Build history of the part. All positions in model axes, mm. A direction names the side the tool comes from. Give positions to 0.01 mm unless a question says otherwise; leave off trailing zeros. Loops run counter-clockwise (first coordinate to the right, second up) from the corner with the lowest first, then second, coordinate; pieces in that order, holes last. Notation, with made-up numbers: (-33, 75) -> (14, 75) arc R22 ccw to (14, 83) -> close; hole circle Ø4 at (44.25, -19.75). An arc over 180 degrees is marked (long way). One line per question, with ' | ' between items. Start each with the question number.
(1) Slice it at C-C, the plane y = 207.5. Write the cut outline in (x, z), then the cut area to 3 significant figures.
(2) Slice it at A-A, the plane x = 58. Write the cut outline in (y, z) (3 decimals), then the cut area to 3 significant figures.
(3) Slice it at B-B, the plane y = 156. Write the cut outline in (x, z) (3 decimals).
(4) Flat gauge pins, fed straight in: pin 1 Ø1.9 at (y, z) = (125, 182) entering from -X; pin 2 Ø10 at (x, y) = (158, 26.5) entering from +Z; pin 3 Ø6 at (x, z) = (95.5, 20) entering from -Y. Where does each tip first touch, or does it go through?
(5) Mould opens along Z. For faces 1 (the face through (90, 223.52, 88)), 2 (the face through (50, 112, 184.15)), 3 (the face through (50, 165.1, 178)) say: pulls with the +Z half, pulls with the -Z half, needs draft (parallel to the pull), parting line crosses it, or undercut.
(6) Drill centre lines: L1, parallel to Y at x = 27, z = 175.5 (3 decimals); L2, parallel to Z at x = 62, y = 190. Where is each one in solid material? Low to high. Write a range as from..to.
(7) 3-axis set-ups, long thin cutter, end or side, ignore diameter. For faces 4 (the face through (172.72, 98, 88)), 5 (the face through (51, 114.3, 178)), 6 (the face through (152.4, 216, 90)): which of +Z, -Z, +X, -X, +Y, -Y reach the whole face in a straight line?
(8) Slice it at D-D, the plane z = 120.5. Write the cut outline in (x, y).
Autodesk Inventor part; units mm, degrees
ref_plane "YZ Plane" through (0, 0, 0) normal (1, 0, 0) x (0, 1, 0)
ref_plane "XZ Plane" through (0, 0, 0) normal (0, 1, 0) x (-1, 0, 0)
ref_plane "XY Plane" through (0, 0, 0) normal (0, 0, 1) x (1, 0, 0)
sketch "Sketch1" plane through (0, 0, 0) normal (0, 0, 1) x (1, 0, 0)
  line L0 (0, 0) -> (177.8, 0)
  line L1 (177.8, 0) -> (177.8, 203.2)
  line L2 (177.8, 203.2) -> (0, 203.2)
  line L3 (0, 203.2) -> (0, 0)
  line L4 (0, 203.2) -> (25.4, 203.2) construction
  line L5 (177.8, 203.2) -> (203.2, 203.2) construction
  line L6 (0, 203.2) -> (177.8, 203.2)
  line L7 (177.8, 203.2) -> (177.8, 228.6)
  line L8 (177.8, 228.6) -> (0, 228.6)
  line L9 (0, 228.6) -> (0, 203.2)
  dimension "d0" = 177.8
  dimension "d1" = 203.2
  dimension "d6" = 177.8
  dimension "d7" = 25.4
extrude "Extrusion1" add sketch "Sketch1" along normal blind 177.8
sketch "Sketch2" plane through (0, 0, 177.8) normal (0, 0, 1) x (1, 0, 0)
  line L0 (177.8, 228.6) -> (0, 228.6)
  line L1 (0, 228.6) -> (177.8, 228.6)
  line L2 (177.8, 228.6) -> (177.8, 203.2)
  line L3 (177.8, 203.2) -> (0, 203.2)
  line L4 (0, 203.2) -> (0, 228.6)
  point P0 (0, 0)
  dimension "d10" = 177.8
  dimension "d11" = 25.4
extrude "Extrusion2" cut sketch "Sketch2" against normal blind 25.4
sketch "Sketch3" plane through (177.8, 0, 0) normal (1, 0, 0) x (0, 0, -1)
  line L0 (0, 0) -> (0, 228.6)
  line L1 (-177.8, 0) -> (-177.8, 203.2)
  line L2 (0, 228.6) -> (-177.8, 228.6)
  line L3 (-177.8, 228.6) -> (-177.8, 203.2)
  line L4 (-177.8, 203.2) -> (0, 203.2)
  line L5 (0, 203.2) -> (0, 228.6)
  dimension "d14" = 177.8
  dimension "d15" = 25.4
extrude "Extrusion3" cut sketch "Sketch3" against normal blind 25.4
sketch "Sketch4" plane through (0, 0, 0) normal (0, 0, -1) x (-1, 0, 0)
  line L0 (0, 228.6) -> (0, 0)
  line L1 (-152.4, 203.2) -> (-177.8, 203.2)
  line L2 (0, 228.6) -> (-177.8, 228.6)
  line L3 (-177.8, 228.6) -> (-177.8, 203.2)
  line L4 (-177.8, 203.2) -> (0, 203.2)
  line L5 (0, 203.2) -> (0, 228.6)
  dimension "d18" = 177.8
  dimension "d19" = 25.4
extrude "Extrusion4" cut sketch "Sketch4" against normal blind 25.4
sketch "Sketch5" plane through (0, 0, 0) normal (-1, 0, 0) x (0, 0, 1)
  line L0 (177.8, 228.6) -> (0, 228.6)
  line L1 (0, 228.6) -> (0, 203.2)
  line L2 (0, 203.2) -> (177.8, 203.2)
  line L3 (177.8, 203.2) -> (177.8, 228.6)
  line L4 (177.8, 203.2) -> (177.8, 0)
  line L5 (25.4, 228.6) -> (152.4, 228.6)
  point P0 (0, 0)
  dimension "d22" = 177.8
  dimension "d23" = 25.4
  dimension "d24" = 0
  dimension "d25" = 0
extrude "Extrusion5" cut sketch "Sketch5" against normal blind 25.4
shell "Shell1" thickness 5.08 removed faces 1 at (59.2667, 0, 59.2667)
sketch "Sketch6" plane through (0, 0, 177.8) normal (0, 0, 1) x (1, 0, 0)
  line L0 (25.4, 165.1) -> (76.2, 165.1)
  line L1 (76.2, 165.1) -> (76.2, 114.3)
  line L2 (76.2, 114.3) -> (25.4, 114.3)
  line L3 (25.4, 114.3) -> (25.4, 165.1)
  line L4 (177.8, 203.2) -> (0, 203.2)
  line L5 (0, 203.2) -> (0, 0)
  line L6 (47.625, 165.1) -> (53.975, 165.1)
  line L7 (53.975, 114.3) -> (47.625, 114.3)
  line L8 (76.2, 142.875) -> (76.2, 136.525)
  line L9 (25.4, 136.525) -> (25.4, 142.875)
  line L10 (47.625, 114.3) -> (47.625, 136.525)
  line L11 (47.625, 142.875) -> (47.625, 165.1)
  line L12 (25.4, 142.875) -> (47.625, 142.875)
  line L13 (53.975, 142.875) -> (76.2, 142.875)
  line L14 (53.975, 165.1) -> (53.975, 142.875)
  line L15 (53.975, 136.525) -> (53.975, 114.3)
  line L16 (76.2, 136.525) -> (53.975, 136.525)
  line L17 (47.625, 136.525) -> (25.4, 136.525)
  line L18 (82.55, 171.45) -> (19.05, 171.45)
  line L19 (19.05, 171.45) -> (19.05, 107.95)
  line L20 (19.05, 107.95) -> (82.55, 107.95)
  line L21 (82.55, 107.95) -> (82.55, 171.45)
  dimension "d29" = 50.8
  dimension "d30" = 50.8
  dimension "d31" = 38.1
  dimension "d32" = 25.4
  dimension "d33" = 6.35
  dimension "d34" = 50.8
  dimension "d36" = 50.8
  dimension "d37" = 6.35
  dimension "d39" = 6.35
extrude "Extrusion6" cut sketch "Sketch6" against normal blind 25.4 contours L0 L11 L12 L3 | L0 L1 L13 L14 | L17 L10 L2 L3 | L1 L2 L15 L16
extrude "Extrusion7" add sketch "Sketch6" along normal blind 6.35
sketch "Sketch7" plane through (0, 0, 177.8) normal (0, 0, 1) x (1, 0, 0)
  line L0 (0, 0) -> (177.8, 0)
  line L1 (76.2, 0) -> (139.7, 0)
  line L2 (139.7, 0) -> (139.7, 88.9)
  line L3 (139.7, 88.9) -> (76.2, 88.9)
  line L4 (76.2, 88.9) -> (76.2, 0)
  line L5 (177.8, 0) -> (177.8, 203.2)
  line L6 (76.2, 0) -> (76.2, 63.5)
  arc A0 (139.7, 63.5) -> (76.2, 63.5) centre (107.95, 56.3852) ccw
  dimension "d44" = 63.5
  dimension "d45" = 88.9
  dimension "d46" = 38.1
  dimension "d47" = 63.5
  dimension "d48" = 32.5374
extrude "Extrusion8" cut sketch "Sketch7" against normal blind 6.35 contours L4 A0 L3 L2 L0 | A0 L3
properties part number "House Model"
Final values:
1) outline: (25.4, 25.4) -> (152.4, 25.4) -> (152.4, 152.4) -> (25.4, 152.4) -> close; hole (30.48, 30.48) -> (147.32, 30.48) -> (147.32, 147.32) -> (30.48, 147.32) -> close | area: 2,480 mm2
2) outline: (0, 0) -> (203.2, 0) -> (203.2, 25.4) -> (228.6, 25.4) -> (228.6, 152.4) -> (203.2, 152.4) -> (203.2, 177.8) -> (171.45, 177.8) -> (171.45, 184.15) -> (165.1, 184.15) -> (165.1, 172.72) -> (198.12, 172.72) -> (198.12, 147.32) -> (223.52, 147.32) -> (223.52, 30.48) -> (198.12, 30.48) -> (198.12, 5.08) -> (0, 5.08) -> close; (0, 172.72) -> (114.3, 172.72) -> (114.3, 184.15) -> (107.95, 184.15) -> (107.95, 177.8) -> (0, 177.8) -> close; (136.525, 172.72) -> (142.875, 172.72) -> (142.875, 177.8) -> (136.525, 177.8) -> close | area: 3,030 mm2
3) outline: (0, 0) -> (177.8, 0) -> (177.8, 177.8) -> (82.55, 177.8) -> (82.55, 184.15) -> (76.2, 184.15) -> (76.2, 172.72) -> (172.72, 172.72) -> (172.72, 5.08) -> (5.08, 5.08) -> (5.08, 172.72) -> (25.4, 172.72) -> (25.4, 184.15) -> (19.05, 184.15) -> (19.05, 177.8) -> (0, 177.8) -> close; (47.625, 172.72) -> (53.975, 172.72) -> (53.975, 177.8) -> (47.625, 177.8) -> close
4) pin 1: x = 19.05 | pin 2: z = 177.8 | pin 3: y = 198.12
5) face 1: undercut | face 2: pulls with the +Z half | face 3: needs draft
6) L1: 0..114.3, 136.525..142.875, 165.1..203.2 | L2: 0..5.08, 172.72..177.8
7) face 4: -Y | face 5: +Z | face 6: +Z, -Z, +X, +Y
8) outline: (0, 0) -> (5.08, 0) -> (5.08, 198.12) -> (30.48, 198.12) -> (30.48, 223.52) -> (147.32, 223.52) -> (147.32, 198.12) -> (172.72, 198.12) -> (172.72, 0) -> (177.8, 0) -> (177.8, 203.2) -> (152.4, 203.2) -> (152.4, 228.6) -> (25.4, 228.6) -> (25.4, 203.2) -> (0, 203.2) -> close
